Can you work these out from the model? Positions are in its coordinate system, mm. Face numbers are marked on the shaded views. A direction names the side the tool comes from. Round coordinates to 2 decimals unless told otherwise and drop trailing zeros. Order: outer loops, then holes, each group sorted by start corner. A loop starts at its lowest first (then second) coordinate and runs counter-clockwise, first axis right, second up. Notation, with made-up numbers: (45.5, 70) -> (90.5, 70) arc R27 ccw to (90.5, 109) -> close; hole circle Ø10 at (-21, 4.5). An arc over 180 degrees is marked (long way). One line per item, written item: value.
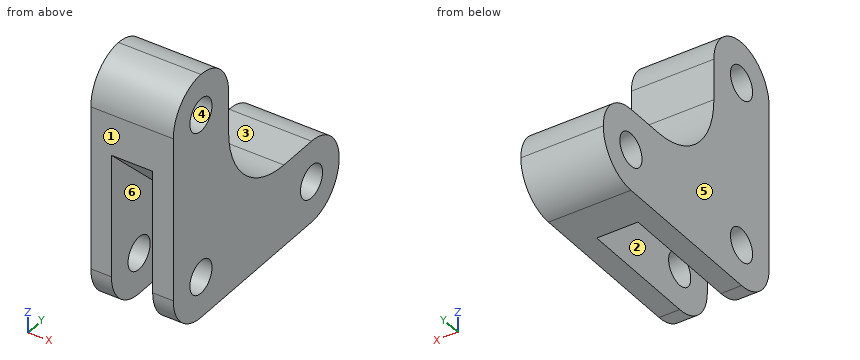
```python
from build123d import *

# Parameters (mm, degrees)
SKETCH1_W           = 10
SKETCH1_H           = 30
BOSS_EXTRUDE1_DEPTH = 10
SKETCH2_W           = 10
SKETCH2_H           = 10
BOSS_EXTRUDE2_DEPTH = 20
SKETCH3_R           = 2
CUT_EXTRUDE1_DEPTH  = 36
FILLET1_R           = 5
FILLET2_R           = 10
SKETCH6_W           = 5
SKETCH6_H           = 10
CUT_EXTRUDE3_DEPTH  = 10
CHAMFER1_SIZE       = 10
SKETCH4_R           = 2
CUT_EXTRUDE4_DEPTH  = 36
FILLET3_R           = 5


with BuildPart() as part:
    # Sketch1 → Boss-Extrude1 (new body)
    with BuildSketch(Plane(origin=(0, 0, 0), x_dir=(1, 0, 0), z_dir=(0, 1, 0))):
        Rectangle(SKETCH1_W, SKETCH1_H)
    extrude(amount=BOSS_EXTRUDE1_DEPTH)

    # Sketch2 → Boss-Extrude2 (add)
    with BuildSketch(Plane(origin=(0, 10, 0), x_dir=(1, 0, 0), z_dir=(0, 1, 0))):
        with Locations((0, 10)):
            Rectangle(SKETCH2_W, SKETCH2_H)
    extrude(amount=BOSS_EXTRUDE2_DEPTH)

    # Sketch3 → Cut-Extrude1 (cut, through all)
    with BuildSketch(Plane(origin=(5, 0, 0), x_dir=(0, 0, -1), z_dir=(1, 0, 0))):
        with Locations((-10, 5)):
            Circle(SKETCH3_R)
        with Locations((10, 25)):
            Circle(SKETCH3_R)
    extrude(amount=-CUT_EXTRUDE1_DEPTH, mode=Mode.SUBTRACT)

    # Fillet1
    fillet1_edges = [part.edges().sort_by_distance(p)[0] for p in [
        (0, 30, -15),
        (0, 30, -5),
        (0, 0, 15),
        (0, 10, 15),
    ]]
    fillet(fillet1_edges, radius=FILLET1_R - 0.0001)  # a hair under: the kernel refuses the full size

    # Fillet2
    fillet2_edges = [part.edges().sort_by_distance(p)[0] for p in [
        (0, 10, -5),
    ]]
    fillet(fillet2_edges, radius=FILLET2_R)

    # Sketch6 → Cut-Extrude3 (cut)
    with BuildSketch(Plane(origin=(0, 0, -15), x_dir=(-1, 0, 0), z_dir=(0, 0, -1))):
        with Locations((0, 5)):
            Rectangle(SKETCH6_W, SKETCH6_H)
    extrude(amount=-CUT_EXTRUDE3_DEPTH, mode=Mode.SUBTRACT)

    # Chamfer1
    chamfer1_edges = [part.edges().sort_by_distance(p)[0] for p in [
        (0, 0, -5),
        (0, 10, -15),
    ]]
    chamfer(chamfer1_edges, length=CHAMFER1_SIZE - 0.0001)  # a hair under: the kernel refuses the full size

    # Sketch4 → Cut-Extrude4 (cut, through all)
    with BuildSketch(Plane(origin=(5, 0, 0), x_dir=(0, 0, -1), z_dir=(1, 0, 0))):
        with Locations((10, 5)):
            Circle(SKETCH4_R)
    extrude(amount=-CUT_EXTRUDE4_DEPTH, mode=Mode.SUBTRACT)

    # Fillet3
    fillet3_edges = [part.edges().sort_by_distance(p)[0] for p in [
        (3.75, 0, -15),
        (-3.75, 0, -15),
    ]]
    fillet(fillet3_edges, radius=FILLET3_R)


solid = part.part
```
Q1. I want a section at A-A on x = -3. Give the number of separate pieces and of enclosed holes in the cut face, plus the area to 3 significant figures.
Answers below:
separate pieces: 1
enclosed holes: 3
area: 457 mm^2
Q2. I want a section at C-C on y = 13.5. List the corners of the cut face in (x, z) for me, plus the area to 3 significant figures.
Answers below:
outline: (-5, -15) -> (-2.5, -15) -> (-2.5, -8.5) -> (2.5, -8.5) -> (2.5, -15) -> (5, -15) -> (5, -2.6) -> (-5, -2.6) -> close
area: 91.5 mm^2
Q3. I want a section at B-B on z = -6.5. List the corners of the cut face in (x, y) for me, plus the area to 3 significant figures.
Answers below:
outline: (-5, 0) -> (-2.5, 0) -> (-2.5, 11.5) -> (2.5, 11.5) -> (2.5, 0) -> (5, 0) -> (5, 28.57) -> (-5, 28.57) -> close
area: 228 mm^2
Q4. Please list where these lines run through material, in increasing order: line 1 along Y through (x, z) = (-3.85, -10); line 2 along X through (y, z) = (3, -12); line 3 along Y through (x, z) = (3.75, -8.5).
Answers below:
line 1: 0 to 3, 7 to 23, 27 to 30
line 2: -5 to -2.5, 2.5 to 5
line 3: 0 to 3.68, 6.32 to 23.68, 26.32 to 29.77
Q5. On a 3-axis mill with a long thin cutter (end or side, diameter ignored), from which of +Z, -Z, +X, -X, +Y, -Y can I reach the whole of each face in a straight line? I mean the marked faces 1, 2 and 3. Say none if no direction works.
Answers below:
face 1: +Z, -Z, +X, -X, -Y
face 2: -Z, -Y
face 3: +Z, +X, -X, +Y
Q6. We'd pull the mould along X, two halves only. Please class the marked faces 4, 5 and 6: released by +X, released by -X, zero draft, split by the parting line, or undercut.
Answers below:
face 4: zero draft
face 5: released by -X
face 6: undercut
Q7. Will these pins go through, and if not, where does the flat tip stop? pin 1 Ø5 at (x, z) = (4, -4.5) entering from +Y; pin 2 Ø12 at (y, z) = (11, 2.5) entering from -X; pin 3 Ø1 at (x, z) = (-3, 11) entering from -Y; pin 4 Ø5 at (x, y) = (2.5, 21.5) entering from +Z.
Answers below:
pin 1: y = 29
pin 2: x = -5
pin 3: y = 0.03
pin 4: z = -4.95
